Here's how the part is built. I have some questions about the finished solid (model axes, mm). Coordinates: 2 decimals unless noted, no trailing zeros. Loops run counter-clockwise (first coordinate to the right, second up) from the corner with the lowest first, then second, coordinate; pieces in that order, holes last. Notation, with made-up numbers: (8, 20.5) -> (28, 20.5) arc R22 ccw to (28, 49.5) -> close; hole circle Ø4 at (87.25, 3.25). An arc over 180 degrees is marked (long way). Answer as a JSON object with one key per item and string values. Group by question number.
Q1. I need wall thicknesses on line 1 (X direction, y = 311, z = -8) (3 decimals); line 2 (Y direction, x = 10.2, z = 0). Which ranges of each line are inside material? Lowest first, please.
Q2. I want a section at B-B on y = 115. Write out the boundary of the cut face in (x, z) (3 decimals).
Q3. I'm going to push a flat-ended pin straight in: pin 1 (5 mm diameter, centred on y = 489.13, z = 0, fed in from -X). Where does the tip first touch, or does it pass through?
Q4. I want a section at A-A on x = 4.5. Write out the boundary of the cut face in (y, z) (3 decimals).
Autodesk Inventor part; units mm, degrees
ref_plane "YZ Plane" through (0, 0, 0) normal (1, 0, 0) x (0, 1, 0)
ref_plane "XZ Plane" through (0, 0, 0) normal (0, 1, 0) x (-1, 0, 0)
ref_plane "XY Plane" through (0, 0, 0) normal (0, 0, 1) x (1, 0, 0)
sketch "Sketch1" plane through (0, 0, 0) normal (0, 1, 0) x (-1, 0, 0)
  line L0 (-12.7, -12.7) -> (12.7, -12.7)
  line L1 (12.7, -12.7) -> (12.7, 12.7)
  line L2 (12.7, 12.7) -> (-12.7, 12.7)
  line L3 (-12.7, 12.7) -> (-12.7, -12.7)
  line L4 (-12.7, -12.7) -> (12.7, 12.7) construction
  line L5 (12.7, -12.7) -> (-12.7, 12.7) construction
  line L6 (-9.525, -9.525) -> (9.525, -9.525)
  line L7 (9.525, -9.525) -> (9.525, 9.525)
  line L8 (9.525, 9.525) -> (-9.525, 9.525)
  line L9 (-9.525, 9.525) -> (-9.525, -9.525)
  line L10 (-9.525, -9.525) -> (9.525, 9.525) construction
  line L11 (9.525, -9.525) -> (-9.525, 9.525) construction
  point P0 (0, 0)
  dimension "d0" = 25.4
  dimension "d1" = 25.4
  dimension "d2" = 19.05
  dimension "d3" = 19.05
extrude "Extrusion1" add sketch "Sketch1" along normal blind 533.4
sketch "Sketch2" plane through (12.7, 0, 12.7) normal (1, 0, 0) x (0, 0, -1)
  line L0 (25.4, 0) -> (25.4, 533.4)
  line L1 (0, 533.4) -> (25.4, 533.4)
  line L2 (0, 533.4) -> (25.4, 508)
  line L3 (0, 533.4) -> (35.921, 533.4) construction
  point P0 (12.7, 0)
  dimension "d6" = 45
extrude "Extrusion2" cut sketch "Sketch2" against normal blind 25.4
sketch "Sketch3" plane through (12.7, 0, 12.7) normal (1, 0, 0) x (0, 0, -1)
  line L0 (25.4, 0) -> (25.4, 508)
  line L1 (12.7, 0) -> (12.7, 17.8054)
  circle A0 centre (12.7, 17.8054) radius 2.54
  dimension "d9" = 17.8054
  dimension "d10" = 5.08
extrude "Extrusion3" cut sketch "Sketch3" against normal blind 25.4
sketch "Sketch4" plane through (12.7, 0, 12.7) normal (1, 0, 0) x (0, 0, -1)
  line L0 (25.4, 0) -> (25.4, 508)
  line L1 (12.7, 0) -> (12.7, 463.7278)
  line L2 (12.7, 0) -> (476.4278, 0) construction
  line L3 (12.7, 463.7278) -> (12.7, 489.1278)
  circle A0 centre (12.7, 489.1278) radius 3.175
  circle A1 centre (12.7, 463.7278) radius 3.175
  dimension "d13" = 463.7278
  dimension "d14" = 90
  dimension "d15" = 25.4
  dimension "d16" = 180
  dimension "d17" = 6.35
  dimension "d18" = 6.35
extrude "Extrusion4" cut sketch "Sketch4" against normal blind 25.4
properties part number "TestSupport"
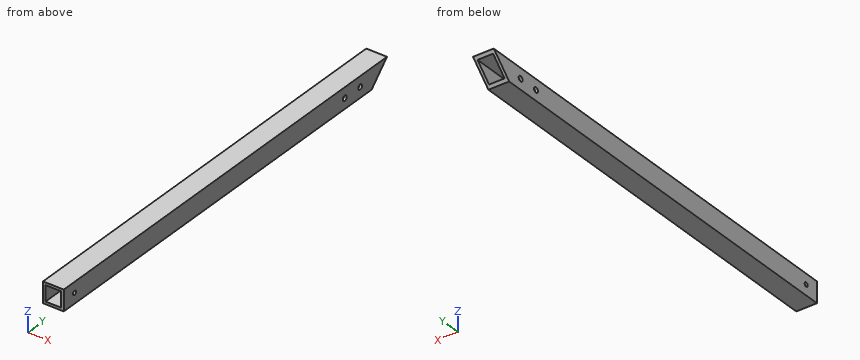
Result set:
{
 "1": {"line 1": "x = -12.7 to -9.525, 9.525 to 12.7", "line 2": "y = 0 to 15.27, 20.35 to 460.55, 466.9 to 485.95, 492.3 to 520.7"},
 "2": {"outline": "(-12.7, -12.7) -> (12.7, -12.7) -> (12.7, 12.7) -> (-12.7, 12.7) -> close; hole (-9.525, -9.525) -> (9.525, -9.525) -> (9.525, 9.525) -> (-9.525, 9.525) -> close"},
 "3": {"pin 1": "passes through"},
 "4": {"outline": "(0, -12.7) -> (508, -12.7) -> (511.175, -9.525) -> (0, -9.525) -> close; (0, 9.525) -> (530.225, 9.525) -> (533.4, 12.7) -> (0, 12.7) -> close"}
}
